from build123d import *

# Parameters (mm, degrees)
EXTRUDE_1_DEPTH     = 14.5
SKETCH_2_W          = 10
SKETCH_2_H          = 3
CUT_EXTRUDE_1_DEPTH = 53.299617589
SKETCH_3_R          = 4
CUT_EXTRUDE_3_DEPTH = 40
FILLET_1_R          = 2
FILLET_2_R          = 2
FILLET_3_R          = 2
FILLET_4_R          = 2
FILLET_5_R          = 2
FILLET_6_R          = 2
SKETCH_5_W          = 6
SKETCH_5_H          = 14.5
EXTRUDE_2_DEPTH     = 4.5
SKETCH_6_W          = 2.5
SKETCH_6_H          = 6
CUT_EXTRUDE_4_DEPTH = 43.026777178


with BuildPart() as part:
    # Эскиз1 → Бобышка-Вытянуть1 (new body)
    with BuildSketch(Plane(origin=(0, 0, 0), x_dir=(1, 0, 0), z_dir=(0, 1, 0))):
        Polygon((0, 0), (-2, 0), (-2, 32), (17, 32), (17, 37), (32, 37), (32, 32), (34, 32), (34, 0), (32, 0), (32, 30), (0, 30), align=None)
    extrude(amount=EXTRUDE_1_DEPTH)

    # Эскиз2 → Вырез-Вытянуть1 (cut, through all)
    with BuildSketch(Plane(origin=(0, 14.5, 0), x_dir=(1, 0, 0), z_dir=(0, 1, 0))):
        with Locations((24.5, 33.5)):
            Rectangle(SKETCH_2_W, SKETCH_2_H)
    extrude(amount=-CUT_EXTRUDE_1_DEPTH, mode=Mode.SUBTRACT)

    # Эскиз3 → Вырез-Вытянуть3 (cut)
    with BuildSketch(Plane(origin=(34, 0, 0), x_dir=(0, 0, -1), z_dir=(1, 0, 0))):
        with Locations((8, 7.25)):
            Circle(SKETCH_3_R)
    extrude(amount=-CUT_EXTRUDE_3_DEPTH, mode=Mode.SUBTRACT)

    # Скругление1
    fillet_1_edges = [part.edges().sort_by_distance(p)[0] for p in [
        (34, 7.25, -32),
    ]]
    fillet(fillet_1_edges, radius=FILLET_1_R - 0.0001)  # a hair under: the kernel refuses the full size

    # Скругление2
    fillet_2_edges = [part.edges().sort_by_distance(p)[0] for p in [
        (-2, 7.25, -32),
    ]]
    fillet(fillet_2_edges, radius=FILLET_2_R)

    # Скругление3
    fillet_3_edges = [part.edges().sort_by_distance(p)[0] for p in [
        (-1, 14.5, 0),
    ]]
    fillet(fillet_3_edges, radius=FILLET_3_R)

    # Скругление4
    fillet_4_edges = [part.edges().sort_by_distance(p)[0] for p in [
        (33, 14.5, 0),
    ]]
    fillet(fillet_4_edges, radius=FILLET_4_R)

    # Скругление5
    fillet_5_edges = [part.edges().sort_by_distance(p)[0] for p in [
        (33, 0, 0),
    ]]
    fillet(fillet_5_edges, radius=FILLET_5_R)

    # Скругление6
    fillet_6_edges = [part.edges().sort_by_distance(p)[0] for p in [
        (-1, 0, 0),
    ]]
    fillet(fillet_6_edges, radius=FILLET_6_R)

    # Эскиз5 → Бобышка-Вытянуть2 (add)
    with BuildSketch(Plane.ZY.offset(2)):
        with Locations((-20, 7.25)):
            Rectangle(SKETCH_5_W, SKETCH_5_H)
    extrude(amount=EXTRUDE_2_DEPTH)

    # Эскиз6 → Вырез-Вытянуть4 (cut, through all)
    with BuildSketch(Plane.XY.offset(-17)):
        with Locations((-3.25, 7.25)):
            Rectangle(SKETCH_6_W, SKETCH_6_H)
    extrude(amount=-CUT_EXTRUDE_4_DEPTH, mode=Mode.SUBTRACT)


solid = part.part
Geometry check sheet. Reference: the model listing, model coordinates, mm. A direction names the side the tool comes from. Coordinates: 2 decimals unless noted, no trailing zeros. Order: outer loops, then holes, each group sorted by start corner. A loop starts at its lowest first (then second) coordinate and runs counter-clockwise, first axis right, second up. Notation, with made-up numbers: (29, 41) -> (73, 41) arc R19 cw to (73, 52) -> close; hole circle Ø4 at (39, 50). An arc over 180 degrees is marked (long way). Use a Markdown table: item, result. Add a question column.
1. Cross-section at D-D (z = -17.5). Enter the section's corners in (x, y).
2. Cross-section at C-C (z = -8). Enter the section's corners in (x, y), and give its area (3 significant figures).
3. Mould release check, pull along Y, two halves, no side actions. Record for faces 4 (the face through (32.99, 13.93, -0.6)), 5 (the face through (-4.5, 7, -20)), 6 (the face through (-3, 10.25, -20)), 7 (the face through (16, 7, -30)): pulls with the +Y half, pulls with the -Y half, needs draft (parallel to the pull), parting line crosses it, or undercut.
4. Cross-section at A-A (z = -33). Enter the section's corners in (x, y), and give its area (3 significant figures).
5. Cross-section at B-B (y = 7.25). Give the number of separate pieces and of enclosed holes in the cut face, and give its area (3 significant figures).
6. Material ranges on L1, parallel to Y at x = -0.4, z = -8; L2, parallel to X at y = 8.75, z = -21; L3, parallel to X at y = 1.5, z = -21.5, recorded low to high.
7. Go/stop test with flat-tipped pins: pin 1 Ø6 at (x, y) = (9, 3) entering from +Z; pin 2 Ø1.3 at (x, y) = (-4, 10.5) entering from -Z; pin 3 Ø5.5 at (y, z) = (9.5, -34.5) entering from +X. Record where each tip stops, or that it passes through.
8. Set-up check for faces 1 (the face through (8, 7, -32)), 2 (the face through (-3, 4.25, -20)), 3 (the face through (-5, 7, -17)): record each of +Z, -Z, +X, -X, +Y, -Y from which the full face is reachable in a straight line by a thin tool's end or side.
Filled sheet:
| question | item | result |
|---|---|---|
| 1 | outline | (-6.5, 0) -> (0, 0) -> (0, 14.5) -> (-6.5, 14.5) -> close; (32, 0) -> (34, 0) -> (34, 14.5) -> (32, 14.5) -> close; hole (-4.5, 4.25) -> (-2, 4.25) -> (-2, 10.25) -> (-4.5, 10.25) -> close |
| 2 | outline | (-2, 0) -> (0, 0) -> (0, 3.25) -> (-2, 3.25) -> close; (-2, 11.25) -> (0, 11.25) -> (0, 14.5) -> (-2, 14.5) -> close; (32, 0) -> (34, 0) -> (34, 3.25) -> (32, 3.25) -> close; (32, 11.25) -> (34, 11.25) -> (34, 14.5) -> (32, 14.5) -> close |
| 2 | area | 26.0 mm2 |
| 3 | face 4 | pulls with the +Y half |
| 3 | face 5 | undercut |
| 3 | face 6 | undercut |
| 3 | face 7 | needs draft |
| 4 | outline | (17, 0) -> (19.5, 0) -> (19.5, 14.5) -> (17, 14.5) -> close; (29.5, 0) -> (32, 0) -> (32, 14.5) -> (29.5, 14.5) -> close |
| 4 | area | 72.5 mm2 |
| 5 | separate pieces | 4 |
| 5 | enclosed holes | 1 |
| 5 | area | 215 mm2 |
| 6 | L1 | 0 to 3.25, 11.25 to 14.5 |
| 6 | L2 | -6.5 to -4.5, -2 to 0, 32 to 34 |
| 6 | L3 | -6.5 to 0, 32 to 34 |
| 7 | pin 1 | z = -30 |
| 7 | pin 2 | z = -23 |
| 7 | pin 3 | x = 32.97 |
| 8 | face 1 | -Z, -X, +Y, -Y |
| 8 | face 2 | +Z, -Z |
| 8 | face 3 | +Z, -X, +Y, -Y |
